Geometry check sheet. Reference: the model listing, model coordinates, mm. A direction names the side the tool comes from. Round coordinates to 2 decimals unless told otherwise and drop trailing zeros. Loops run counter-clockwise (first coordinate to the right, second up) from the corner with the lowest first, then second, coordinate; pieces in that order, holes last. Notation, with made-up numbers: M 87,-25.5 L 106,-25.5 A12 ccw 106,-16.5 Z; hole C 84.5,82.5 d2. An arc over 180 degrees is marked long. Use one line per item in the form item = value. Start each with the question number.
1. Cross-section at C-C (y = 17). Record the boundary of the cut face in (x, z) (3 decimals).
2. Set-up check for faces 1 (the flat face through (0, 0, -6.985)), 2 (the flat face through (2, 1, -13.335)): record each of +Z, -Z, +X, -X, +Y, -Y from which the full face is reachable in a straight line by a thin tool's end or side.
3. Cross-section at B-B (y = 26.5). Record the boundary of the cut face in (x, z) (3 decimals), then the cut area to 3 significant figures.
4. Go/stop test with flat-tipped pins: pin 1 (12 mm diameter, centred on x = -7, y = 25.5, fed in from +Z); pin 2 (4.5 mm diameter, centred on x = 21, z = -2, fed in from -Y); pin 3 (2 mm diameter, centred on x = 32.5, z = -5.5, fed in from +Y) (3 decimals); pin 4 (12 mm diameter, centred on x = 12, z = -3, fed in from -Y) (3 decimals). Record where each tip stops, or that it passes through.
5. Draft check along Y on faces 3 (the cylindrical face through (-5.08, -0.03, -8.96)), 4 (the flat face through (22, -3.175, -6)), 5 (the cylindrical face through (4.39, -1.38, -12.83)), 6 (the flat face through (-13.752, 17.468, -6.37)). Enter one of: pulls with the +Y half, pulls with the -Y half, needs draft (parallel to the pull), parting line crosses it, or undercut.
6. Material ranges on line 1 (Y direction, x = 0, z = -12.5); line 2 (Y direction, x = 0, z = -9.4), recorded low to high.
7. Cross-section at A-A (z = -3). State how many separate pieces and enclosed holes the cut face has, then the cut area to 3 significant figures.
```python
from build123d import *

# Parameters (mm, degrees)
F1_DEPTH  = 3.175
F3_DEPTH  = 10.16
F5_DEPTH  = 19.2661186822
F6_COUNT  = 3
F8_DEPTH  = 6.85
F9_R      = 4.6025
F9_R_2    = 2.0625
F10_DEPTH = 1


with BuildPart() as f1:
    # F0 (on Front) → F1 (new body, symmetric)
    with BuildSketch(Plane.XZ):
        Polygon((0, -5.485), (0, -6.985), (2.0625, -6.985), (2.0625, -12.335), (30.8073278059, -12.335), (46.8930374778, -1.2901832047), (41.1420940815, 7.0855107996), (33.7226801014, 1.9911711769), (22.8343583448, -5.485), align=None)
    extrude(amount=F1_DEPTH, both=True)

    # F2 (on face) → F3 (join, through all)
    with BuildSketch(Plane(origin=(9.8755636575, 0, -14.3828053272), x_dir=(0.8243793311, 0, 0.5660377358), z_dir=(-0.5660377358, 0, 0.8243793311))):
        with BuildLine():
            Line((30.23841274, 3.175), (36.6163042411, 3.175))
            ThreePointArc((36.6163042411, 3.175), (33.4273584906, 4.5), (30.23841274, 3.175))
        make_face()
        with BuildLine():
            ThreePointArc((30.23841274, -3.175), (33.4273584906, -4.5), (36.6163042411, -3.175))
            Line((36.6163042411, -3.175), (30.23841274, -3.175))
        make_face()
        with BuildLine():
            ThreePointArc((36.6163042411, -3.175), (37.5867007389, -1.7175191589), (37.9273584906, 0))
            ThreePointArc((37.9273584906, 0), (37.5867007389, 1.7175191589), (36.6163042411, 3.175))
            Line((36.6163042411, 3.175), (30.23841274, 3.175))
            ThreePointArc((30.23841274, 3.175), (28.9273584906, 0), (30.23841274, -3.175))
            Line((30.23841274, -3.175), (36.6163042411, -3.175))
        make_face()
    extrude(amount=-F3_DEPTH)

    # F4 (on face) → F5 (cut, through all)
    with BuildSketch(Plane(origin=(9.8755636575, 0, -14.3828053272), x_dir=(0.8243793311, 0, 0.5660377358), z_dir=(-0.5660377358, 0, 0.8243793311))):
        with BuildLine():
            Line((36.6163042411, -3.175), (37.9273584906, -3.175))
            Line((37.9273584906, -3.175), (37.9273584906, 0))
            ThreePointArc((37.9273584905, 0), (37.5867007389, -1.7175191589), (36.6163042411, -3.175))
        make_face()
        with BuildLine():
            ThreePointArc((36.6163042411, 3.175), (37.5867007389, 1.7175191589), (37.9273584905, 0))
            Line((37.9273584906, 0), (37.9273584906, 3.175))
            Line((37.9273584906, 3.175), (36.6163042411, 3.175))
        make_face()
    extrude(amount=-F5_DEPTH, mode=Mode.SUBTRACT)

    # F6: F1 ×3 about axis
    f6_axis = Axis((0, 0, -2.7425), (0, 0, -1))


with BuildPart() as f1_1:
    add(f1.part)
    for i in range(1, F6_COUNT):
        add(f1.part.rotate(f6_axis, i * 360 / F6_COUNT))

    # F7 (on face) → F8 (join, through all)
    with BuildSketch(Plane(origin=(0, 0, -12.335), x_dir=(1, 0, 0), z_dir=(0, 0, -1))):
        with BuildLine():
            ThreePointArc((-1.031249974, 1.7861774103), (1.031250013, 1.7861773878), (2.0625, 0))
            Line((2.0625, 0), (2.0625, 3.175))
            Line((2.0625, 3.175), (3.965573729, 3.175))
            ThreePointArc((3.965573729, 3.175), (2.54, 4.3994090512), (0.7668437925, 5.0217875899))
            Line((0.7668437925, 5.0217875899), (1.718380657, 3.3736773953))
            Line((1.718380657, 3.3736773953), (-1.031249974, 1.7861774103))
        make_face()
        with BuildLine():
            Line((2.0625, -3.175), (2.0625, 0))
            ThreePointArc((2.0625, 0), (-1.031250013, -1.7861773878), (-1.031249974, 1.7861774103))
            Line((-1.031249974, 1.7861774103), (-3.780880657, 0.1986773953))
            Line((-3.780880657, 0.1986773953), (-4.7324175215, 1.8467875899))
            ThreePointArc((-4.7324175215, 1.8467875899), (-2.54, -4.3994090512), (3.965573729, -3.175))
            Line((3.965573729, -3.175), (2.0625, -3.175))
        make_face()
    extrude(amount=-F8_DEPTH)

    # F9 (on face) → F10 (join)
    with BuildSketch(Plane(origin=(0, 0, -12.335), x_dir=(1, 0, 0), z_dir=(0, 0, -1))):
        Circle(F9_R)
        Circle(F9_R_2, mode=Mode.SUBTRACT)
    extrude(amount=F10_DEPTH)


solid = f1_1.part
```
Reported:
q1.outline = M -13.481,-12.335 L -6.149,-12.335 L -6.149,-5.485 L -13.481,-5.485 Z
q2.face_1 = -Z
q2.face_2 = -Z, +X, -X, +Y, -Y
q3.outline = M -18.966,-11.219 L -15.715,-12.335 L -11.634,-12.335 L -11.634,-1.412 L -18.966,1.105 Z
q3.area = 87.5 mm²
q4.pin_1 = -0.26
q4.pin_2 = through
q4.pin_3 = 3.175
q4.pin_4 = -3.175
q5.face_3 = undercut
q5.face_4 = pulls with the -Y half
q5.face_5 = parting line crosses it
q5.face_6 = undercut
q6.line_1 = -4.6 to -2.06, 2.06 to 4.6
q6.line_2 = -6.35 to -2.06, 2.06 to 6.35
q7.separate_pieces = 3
q7.enclosed_holes = 0
q7.area = 377 mm²
